Source: CAD feature listing. Evaluate the final solid. Frame: model axes, mm. Round coordinates to 2 decimals unless told otherwise and drop trailing zeros. Loops run counter-clockwise (first coordinate to the right, second up) from the corner with the lowest first, then second, coordinate; pieces in that order, holes last. Notation, with made-up numbers: (43.25, 16) -> (64.25, 16) arc R5 cw to (64.25, 22) -> close; hole circle Ø7 at (32, -26). An arc over 180 degrees is marked (long way). Put each result on its own line as item: value. Start each with the question number.
1. Cut plane A-A (y = 5). Return the cut outline in (x, z).
2. Cut plane B-B (z = -19). Return the cut outline in (x, y).
3. Contact query for flat-ended pins moving along their axis: pin 1 (3 mm diameter, centred on y = 3, z = -29, fed in from +X); pin 2 (1.5 mm diameter, centred on y = 2, z = 18.5, fed in from -X); pin 3 (1 mm diameter, centred on y = 1, z = -19, fed in from +X). Output: stop coordinate, or through.
4. Material intervals for L1, parallel to X at y = 4.75, z = 10.5; L2, parallel to Z at x = 37, y = 3.75; L3, parallel to Z at x = -18, y = 1, sorted ascending.
5. Cut plane C-C (x = 28). Return the cut outline in (y, z), then the cut area to 3 significant figures.
```python
from build123d import *
from OCP.BRepFilletAPI import BRepFilletAPI_MakeChamfer

# Parameters (mm, degrees)
EXTRUDE2_DEPTH     = 8
CHAMFER2_SIZE      = 4
CHAMFER2_SIZE2     = 2.309401077
CUT_EXTRUDE1_DEPTH = 3


with BuildPart() as part:
    # Sketch1 → Extrude2 (new body)
    with BuildSketch(Plane(origin=(0, 0, 0), x_dir=(1, 0, 0), z_dir=(0, 1, 0))):
        with BuildLine():
            Line((-6.5, 41.572883869), (-16.221725084, 16.871170844))
            ThreePointArc((-16.221725084, 16.871170844), (-17.527996386, 13.882959965), (-19.052558883, 11))
            ThreePointArc((-19.052558883, 11), (-20.786994202, 8.238210165), (-22.721725084, 5.612840594))
            Line((-22.721725084, 5.612840594), (-39.253173539, -15.15727681))
            ThreePointArc((-39.253173539, -15.15727681), (-39.837168574, -23), (-32.753173539, -26.415607059))
            Line((-32.753173539, -26.415607059), (-6.5, -22.484011438))
            ThreePointArc((-6.5, -22.484011438), (-3.258997817, -22.12117013), (0, -22))
            ThreePointArc((0, -22), (3.258997817, -22.12117013), (6.5, -22.484011438))
            Line((6.5, -22.484011438), (32.753173539, -26.415607059))
            ThreePointArc((32.753173539, -26.415607059), (39.837168574, -23), (39.253173539, -15.15727681))
            Line((39.253173539, -15.15727681), (22.721725084, 5.612840594))
            ThreePointArc((22.721725084, 5.612840594), (20.786994202, 8.238210165), (19.052558883, 11))
            ThreePointArc((19.052558883, 11), (17.527996386, 13.882959965), (16.221725084, 16.871170844))
            Line((16.221725084, 16.871170844), (6.5, 41.572883869))
            ThreePointArc((6.5, 41.572883869), (0, 46), (-6.5, 41.572883869))
        make_face()
    extrude(amount=EXTRUDE2_DEPTH)

    # Chamfer2: one chamfer whose edges measure the first distance from different faces: ONE call of the kernel's chamfer builder (chamfer() names one face for all edges)
    chamfer2_edges_1 = [part.edges().sort_by_distance(p)[0] for p in [
        (-19.052558883, 8, -11),
    ]]
    chamfer2_side_1 = [part.faces().sort_by_distance(p)[0] for p in [
        (-19.052558883, 4, -11),
    ]]
    chamfer2_edges_2 = [part.edges().sort_by_distance(p)[0] for p in [
        (-30.987449312, 8, 4.772218108),
    ]]
    chamfer2_side_2 = [part.faces().sort_by_distance(p)[0] for p in [
        (-30.987449312, 4, 4.772218108),
    ]]
    chamfer2_edges_3 = [part.edges().sort_by_distance(p)[0] for p in [
        (-39.837168574, 8, 23),
    ]]
    chamfer2_side_3 = [part.faces().sort_by_distance(p)[0] for p in [
        (-39.837168574, 4, 23),
    ]]
    chamfer2_edges_4 = [part.edges().sort_by_distance(p)[0] for p in [
        (-19.626586769, 8, 24.449809248),
    ]]
    chamfer2_side_4 = [part.faces().sort_by_distance(p)[0] for p in [
        (-19.626586769, 4, 24.449809248),
    ]]
    chamfer2_edges_5 = [part.edges().sort_by_distance(p)[0] for p in [
        (0, 8, 22),
    ]]
    chamfer2_side_5 = [part.faces().sort_by_distance(p)[0] for p in [
        (0, 4, 22),
    ]]
    chamfer2_edges_6 = [part.edges().sort_by_distance(p)[0] for p in [
        (19.626586769, 8, 24.449809248),
    ]]
    chamfer2_side_6 = [part.faces().sort_by_distance(p)[0] for p in [
        (19.626586769, 4, 24.449809248),
    ]]
    chamfer2_edges_7 = [part.edges().sort_by_distance(p)[0] for p in [
        (39.837168574, 8, 23),
    ]]
    chamfer2_side_7 = [part.faces().sort_by_distance(p)[0] for p in [
        (39.837168574, 4, 23),
    ]]
    chamfer2_edges_8 = [part.edges().sort_by_distance(p)[0] for p in [
        (30.987449312, 8, 4.772218108),
    ]]
    chamfer2_side_8 = [part.faces().sort_by_distance(p)[0] for p in [
        (30.987449312, 4, 4.772218108),
    ]]
    chamfer2_edges_9 = [part.edges().sort_by_distance(p)[0] for p in [
        (0, 8, -46),
    ]]
    chamfer2_side_9 = [part.faces().sort_by_distance(p)[0] for p in [
        (0, 4, -46),
    ]]
    chamfer2_edges_10 = [part.edges().sort_by_distance(p)[0] for p in [
        (19.052558883, 8, -11),
    ]]
    chamfer2_side_10 = [part.faces().sort_by_distance(p)[0] for p in [
        (19.052558883, 4, -11),
    ]]
    chamfer2_edges_11 = [part.edges().sort_by_distance(p)[0] for p in [
        (11.360862542, 8, -29.222027356),
    ]]
    chamfer2_side_11 = [part.faces().sort_by_distance(p)[0] for p in [
        (11.360862542, 4, -29.222027356),
    ]]
    chamfer2_edges_12 = [part.edges().sort_by_distance(p)[0] for p in [
        (-11.360862542, 8, -29.222027356),
    ]]
    chamfer2_side_12 = [part.faces().sort_by_distance(p)[0] for p in [
        (-11.360862542, 4, -29.222027356),
    ]]
    chamfer2 = BRepFilletAPI_MakeChamfer(part.part.solid().wrapped)
    for e in chamfer2_edges_1:
        chamfer2.Add(CHAMFER2_SIZE, CHAMFER2_SIZE2, e.wrapped, chamfer2_side_1[0].wrapped)  # the first distance lies on this face
    for e in chamfer2_edges_2:
        chamfer2.Add(CHAMFER2_SIZE, CHAMFER2_SIZE2, e.wrapped, chamfer2_side_2[0].wrapped)  # the first distance lies on this face
    for e in chamfer2_edges_3:
        chamfer2.Add(CHAMFER2_SIZE, CHAMFER2_SIZE2, e.wrapped, chamfer2_side_3[0].wrapped)  # the first distance lies on this face
    for e in chamfer2_edges_4:
        chamfer2.Add(CHAMFER2_SIZE, CHAMFER2_SIZE2, e.wrapped, chamfer2_side_4[0].wrapped)  # the first distance lies on this face
    for e in chamfer2_edges_5:
        chamfer2.Add(CHAMFER2_SIZE, CHAMFER2_SIZE2, e.wrapped, chamfer2_side_5[0].wrapped)  # the first distance lies on this face
    for e in chamfer2_edges_6:
        chamfer2.Add(CHAMFER2_SIZE, CHAMFER2_SIZE2, e.wrapped, chamfer2_side_6[0].wrapped)  # the first distance lies on this face
    for e in chamfer2_edges_7:
        chamfer2.Add(CHAMFER2_SIZE, CHAMFER2_SIZE2, e.wrapped, chamfer2_side_7[0].wrapped)  # the first distance lies on this face
    for e in chamfer2_edges_8:
        chamfer2.Add(CHAMFER2_SIZE, CHAMFER2_SIZE2, e.wrapped, chamfer2_side_8[0].wrapped)  # the first distance lies on this face
    for e in chamfer2_edges_9:
        chamfer2.Add(CHAMFER2_SIZE, CHAMFER2_SIZE2, e.wrapped, chamfer2_side_9[0].wrapped)  # the first distance lies on this face
    for e in chamfer2_edges_10:
        chamfer2.Add(CHAMFER2_SIZE, CHAMFER2_SIZE2, e.wrapped, chamfer2_side_10[0].wrapped)  # the first distance lies on this face
    for e in chamfer2_edges_11:
        chamfer2.Add(CHAMFER2_SIZE, CHAMFER2_SIZE2, e.wrapped, chamfer2_side_11[0].wrapped)  # the first distance lies on this face
    for e in chamfer2_edges_12:
        chamfer2.Add(CHAMFER2_SIZE, CHAMFER2_SIZE2, e.wrapped, chamfer2_side_12[0].wrapped)  # the first distance lies on this face
    add(Compound.cast(chamfer2.Shape()), mode=Mode.REPLACE)

    # Sketch2 → Cut-Extrude1 (cut)
    with BuildSketch(Plane(origin=(0, 0, 0), x_dir=(1, 0, 0), z_dir=(0, 1, 0))):
        with BuildLine():
            ThreePointArc((-33.135101254, -24.464580596), (-38.117859233, -22.00735629), (-37.754498914, -16.463549149))
            ThreePointArc((-37.754498914, -16.463549149), (-36.352384156, -16.278957239), (-36.167792243, -17.681071999))
            ThreePointArc((-36.167792243, -17.681071999), (-36.385808436, -21.007356296), (-33.396153637, -22.481690885))
            ThreePointArc((-33.396153637, -22.481690885), (-32.274182592, -23.342609551), (-33.135101254, -24.464580596))
        make_face()
        with BuildLine():
            ThreePointArc((-4.619397662, 40.928129741), (-1e-09, 44.014712579), (4.619397658, 40.928129741))
            ThreePointArc((4.619397658, 40.928129741), (4.078201562, 39.621566787), (2.771638604, 40.162762881))
            ThreePointArc((2.771638604, 40.162762881), (-1e-09, 42.014712591), (-2.771638608, 40.162762881))
            ThreePointArc((-2.771638608, 40.162762881), (-4.078201566, 39.621566787), (-4.619397662, 40.928129741))
        make_face()
        with BuildLine():
            ThreePointArc((37.754498916, -16.463549145), (38.117859234, -22.007356289), (33.135101256, -24.464580593))
            ThreePointArc((33.135101256, -24.464580593), (32.274182594, -23.342609548), (33.396153639, -22.481690882))
            ThreePointArc((33.396153639, -22.481690882), (36.385808436, -21.007356295), (36.167792245, -17.681071996))
            ThreePointArc((36.167792245, -17.681071996), (36.352384158, -16.278957236), (37.754498916, -16.463549145))
        make_face()
    extrude(amount=CUT_EXTRUDE1_DEPTH, mode=Mode.SUBTRACT)


solid = part.part
```
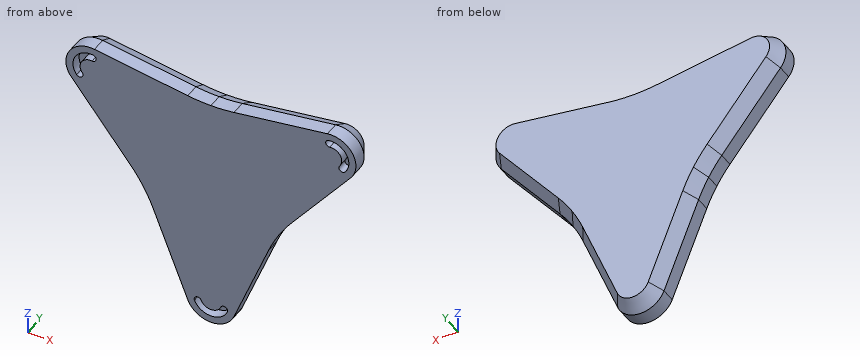
Solution:
1. outline: (-38.8, 15.52) -> (-22.27, -5.25) arc R44.47 cw to (-15.68, -16.66) -> (-5.96, -41.36) arc R6.41 ccw to (5.96, -41.36) -> (15.68, -16.66) arc R44.47 cw to (22.27, -5.25) -> (38.8, 15.52) arc R6.41 ccw to (32.84, 25.84) -> (6.59, 21.91) arc R44.47 cw to (-6.59, 21.91) -> (-32.84, 25.84) arc R6.41 ccw to start
2. outline: (-15.38, 0) -> (15.38, 0) -> (15.38, 4) -> (12.9, 8) -> (-12.9, 8) -> (-15.38, 4) -> close
3. pin 1: stops at x = 12.04
3. pin 2: stops at x = -40.77
3. pin 3: stops at x = 15.58
4. L1: x = -34.99 to 34.99
4. L2: z = 12.33 to 25.71
4. L3: z = -12.93 to 24.21
5. outline: (0, 1.02) -> (4, 1.02) -> (8, 4.73) -> (8, 23.37) -> (4, 25.7) -> (0, 25.7) -> close
5. area: 185 mm^2
